Verification items for the finished model (mm, model axes). Face numbers are marked on the shaded views. A direction names the side the tool comes from. Give positions to 0.01 mm unless a question says otherwise; leave off trailing zeros. Loops run counter-clockwise (first coordinate to the right, second up) from the corner with the lowest first, then second, coordinate; pieces in that order, holes last. Notation, with made-up numbers: M 85.25,-22 L 116.25,-22 A23 cw 116.25,7 Z; hole C -27.75,-28 d5. An arc over 180 degrees is marked long. Answer in a Markdown table with one row per item.
```python
from build123d import *

# Parameters (mm, degrees)
F1_DEPTH = 15
F3_D     = 3
F3_DEPTH = 10
F5_D     = 3
F5_DEPTH = 10
F7_D     = 3
F7_DEPTH = 50


with BuildPart() as f1:
    # F0 (on Front) → F1 (new body)
    with BuildSketch(Plane.XZ):
        with BuildLine():
            Line((-27.360521, 90.12893), (-27.360521, -89.87107))
            ThreePointArc((-27.360521, -89.87107), (-7.360521, -109.87107), (12.639479, -89.87107))
            Line((12.639479, -89.87107), (12.639479, 90.12893))
            Line((12.639479, 90.12893), (9.639479, 90.12893))
            Line((9.639479, 90.12893), (9.639479, -89.87107))
            ThreePointArc((9.639479, -89.87107), (-7.360521, -106.87107), (-24.360521, -89.87107))
            Line((-24.360521, -89.87107), (-24.360521, 90.12893))
            Line((-24.360521, 90.12893), (-27.360521, 90.12893))
        make_face()
    extrude(amount=F1_DEPTH)

    # F3
    with Locations(Plane(origin=(-27.360521, 0, 0), x_dir=(0, -1, 0), z_dir=(-1, 0, 0))):
        with Locations((7.5, 80.12893), (7.5, 20.130026), (7.5, 0.130026), (7.5, -59.869974), (7.5, 60.12893), (7.5, 40.130026), (7.5, -19.869974), (7.5, -39.869974)):
            Hole(F3_D / 2, depth=F3_DEPTH)

    # F5
    with Locations(Plane.YZ.offset(12.639479)):
        with Locations((-7.5, 80.12893), (-7.5, 20.12893), (-7.5, 0.12893), (-7.5, -59.87107)):
            Hole(F5_D / 2, depth=F5_DEPTH)

    # F7
    with Locations(Plane.YZ.offset(12.639479)):
        with Locations((-7.5, -96.87107)):
            Hole(F7_D / 2, depth=F7_DEPTH)


solid = f1.part
```
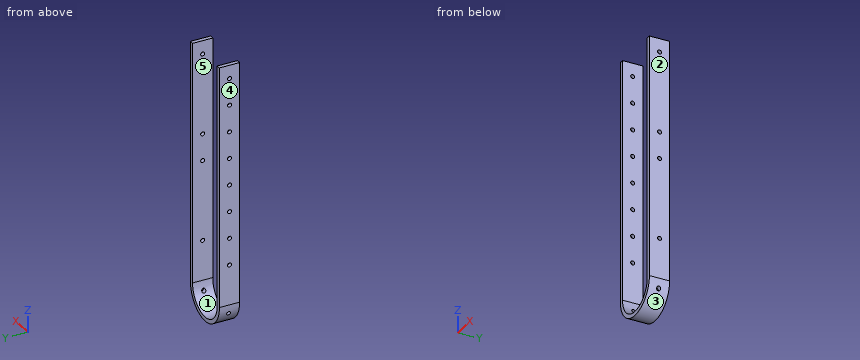
Item 1: Tool access check on the marked faces 4 and 5. Record the directions out of +Z, -Z, +X, -X, +Y, -Y that give a thin tool (end or side, any length) a straight path to the whole face; none if there is none.
Reported:
| item | result |
|---|---|
| face 4 | +Z, -Z, -X, +Y, -Y |
| face 5 | +Z, +Y, -Y |
Item 2: Go/stop test with flat-tipped pins: pin 1 (4 mm diameter, centred on y = -7.5, z = 20.13, fed in from +X); pin 2 (3 mm diameter, centred on x = 3, y = -3.5, fed in from +Z); pin 3 (3.5 mm diameter, centred on y = -7.5, z = -96.87, fed in from -X); pin 4 (2 mm diameter, centred on x = 5, y = -7, fed in from +Z). Record where each tip stops, or that it passes through.
Reported:
| item | result |
|---|---|
| pin 1 | stops at x = 12.64 |
| pin 2 | stops at z = -102.05 |
| pin 3 | stops at x = -26.66 |
| pin 4 | stops at z = -100.38 |
Item 3: Sectioned sample at C-C (x = -2). Record the cut outline in (y, z).
Reported:
| item | result |
|---|---|
| outline | M -15,-109.14 L 0,-109.14 L 0,-106 L -15,-106 Z |
Item 4: Sectioned sample at B-B (y = -12.5). Record the cut outline in (x, z), and give its area (3 significant figures).
Reported:
| item | result |
|---|---|
| outline | M -27.36,-89.87 A20 ccw 12.64,-89.87 L 12.64,90.13 L 9.64,90.13 L 9.64,-89.87 A17 cw -24.36,-89.87 L -24.36,90.13 L -27.36,90.13 Z |
| area | 1,250 mm^2 |
Item 5: Release check for a two-part mould opening along X. For the marked faces 1, 2 and 3 record: released by +X, released by -X, zero draft, split by the parting line, or undercut.
Reported:
| item | result |
|---|---|
| face 1 | undercut |
| face 2 | released by +X |
| face 3 | split by the parting line |
Item 6: Scan lines: L1, parallel to X at y = -9.5, z = 54.5; L2, parallel to Z at x = 10.65, y = -7.5; L3, parallel to Z at x = -8, y = -13. Record each from-to range of solid material in increasing order. Write a range as [from, to].
Reported:
| item | result |
|---|---|
| L1 | x = [-27.36, -24.36], [9.64, 12.64] |
| L2 | z = [-98.57, -98.37], [-95.37, -61.37], [-58.37, -1.37], [1.63, 18.63], [21.63, 78.63], [81.63, 90.13] |
| L3 | z = [-109.86, -106.86] |
Item 7: Sectioned sample at A-A (z = -51). Record the cut outline in (x, y).
Reported:
| item | result |
|---|---|
| outline | M -27.36,-15 L -24.36,-15 L -24.36,0 L -27.36,0 Z; M 9.64,-15 L 12.64,-15 L 12.64,0 L 9.64,0 Z |
Item 8: Sectioned sample at D-D (x = -15). Record the cut outline in (y, z), and give its area (3 significant figures).
Reported:
| item | result |
|---|---|
| outline | M -15,-108.35 L 0,-108.35 L 0,-105.06 L -15,-105.06 Z |
| area | 49.5 mm^2 |
